The model under review builds one solid part; all positions refer to its coordinate system, in mm. A direction names the side the tool comes from. Give positions to 0.01 mm unless a question says otherwise; leave off trailing zeros. Order: outer loops, then holes, each group sorted by start corner. A loop starts at its lowest first (then second) coordinate and runs counter-clockwise, first axis right, second up.
```python
from build123d import *

# Parameters (mm, degrees)
MAIN_DEPTH                 = 20
ESQUISSE2_R                = 1.6
TOPHOLE_DEPTH              = 5
R_P_TITION_LIN_AIRE1_COUNT = 4
R_P_TITION_LIN_AIRE1_PITCH = 10


with BuildPart() as part:
    # Esquisse1 → Main (new body)
    with BuildSketch(Plane.XY):
        Polygon((-5, 0), (-5, 3), (-1.45, 3), (-1.45, 4), (1.45, 4), (1.45, 3), (5, 3), (5, 0), align=None)
    main = extrude(amount=MAIN_DEPTH)

    # Esquisse2 → TopHole (cut, through all)
    with BuildSketch(Plane(origin=(0, 4, 0), x_dir=(1, 0, 0), z_dir=(0, 1, 0))):
        with Locations((0, -5)):
            Circle(ESQUISSE2_R)
        with Locations((0, -15)):
            Circle(ESQUISSE2_R)
    tophole = extrude(amount=-TOPHOLE_DEPTH, mode=Mode.SUBTRACT)

    # Répétition linéaire1: Main, TopHole ×4
    with Locations(*[(-i * R_P_TITION_LIN_AIRE1_PITCH, 0, 0) for i in range(1, R_P_TITION_LIN_AIRE1_COUNT)]):
        add(main)
        add(tophole, mode=Mode.SUBTRACT)


solid = part.part
```
1. To check wall thickness, follow line 1 (X direction, y = 1.8, z = 5); line 2 (Z direction, x = -30, y = 1.25); line 3 (X direction, y = 3.25, z = 9). State the ranges of each line that lie inside material, in increasing order.
2. Take a section at B-B (y = 0.5). Count the separate pieces of the cut face and the enclosed holes in it, and give its area (3 significant figures).
3. For faces 3 (the flat face through (1.45, 3.5, 9.9)), 4 (the flat face through (-1.45, 3.5, 17.8)), 5 (the flat face through (-33, 3, 10)), list the 3-axis set-ups (+Z, -Z, +X, -X, +Y, -Y) from which the entire face can be reached by the end or side of a thin tool; tool diameter is ignored.
4. Insertion check: pin 1 (0.8 mm diameter, centred on y = 3.5, z = 2, fed in from -X); pin 2 (0.8 mm diameter, centred on y = 3.5, z = 17, fed in from +X); pin 3 (3.5 mm diameter, centred on x = -14.5, z = 7, fed in from +Y). Each pin has a flat end and moves straight along its axis. Give the tip position at first contact, or say it passes through.
5. Draft analysis for pull direction Z (two halves, no side actions). For faces 1 (the flat face through (0, 4, 2)), 2 (the cylindrical face through (-1.6, 2.03, 14.93)), state which applies: pulls with the +Z half, pulls with the -Z half, needs draft (parallel to the pull), parting line crosses it, or undercut.
6. Take a section at C-C (z = 5). Write out the cut boundary in (x, y), and give its area (3 significant figures).
7. Take a section at A-A (x = 0). Write out the cut boundary in (y, z).
8. Take a section at D-D (z = 18.75). Write out the cut boundary in (x, y), and give its area (3 significant figures).
Answer:
1. line 1: x = -35 to -31.6, -28.4 to -21.6, -18.4 to -11.6, -8.4 to -1.6, 1.6 to 5
1. line 2: z = 0 to 3.4, 6.6 to 13.4, 16.6 to 20
1. line 3: x = -31.45 to -28.55, -21.45 to -18.55, -11.45 to -8.55, -1.45 to 1.45
2. separate pieces: 1
2. enclosed holes: 8
2. area: 736 mm2
3. face 3: +Z, -Z, +X, +Y
3. face 4: +Z, -Z, +Y
3. face 5: +Z, -Z, -X, +Y
4. pin 1: stops at x = -31.45
4. pin 2: stops at x = 1.45
4. pin 3: stops at y = 3
5. face 1: needs draft
5. face 2: undercut
6. outline: (-35, 0) - (-31.6, 0) - (-31.6, 3) - (-35, 3) - close; (-28.4, 0) - (-21.6, 0) - (-21.6, 3) - (-28.4, 3) - close; (-18.4, 0) - (-11.6, 0) - (-11.6, 3) - (-18.4, 3) - close; (-8.4, 0) - (-1.6, 0) - (-1.6, 3) - (-8.4, 3) - close; (1.6, 0) - (5, 0) - (5, 3) - (1.6, 3) - close
6. area: 81.6 mm2
7. outline: (0, 0) - (4, 0) - (4, 3.4) - (0, 3.4) - close; (0, 6.6) - (4, 6.6) - (4, 13.4) - (0, 13.4) - close; (0, 16.6) - (4, 16.6) - (4, 20) - (0, 20) - close
8. outline: (-35, 0) - (5, 0) - (5, 3) - (1.45, 3) - (1.45, 4) - (-1.45, 4) - (-1.45, 3) - (-8.55, 3) - (-8.55, 4) - (-11.45, 4) - (-11.45, 3) - (-18.55, 3) - (-18.55, 4) - (-21.45, 4) - (-21.45, 3) - (-28.55, 3) - (-28.55, 4) - (-31.45, 4) - (-31.45, 3) - (-35, 3) - close
8. area: 132 mm2
